CAD build for the part. Positions are in the model's coordinates, mm. Coordinates: 2 decimals unless noted, no trailing zeros. Loops run counter-clockwise (first coordinate to the right, second up) from the corner with the lowest first, then second, coordinate; pieces in that order, holes last. Notation, with made-up numbers: (65, 67) -> (84, 67) arc R30 cw to (84, 89) -> close; hole circle Ø3 at (30.25, 44.25). An arc over 180 degrees is marked (long way). Write each question's results on one line, items separated by ' | '.
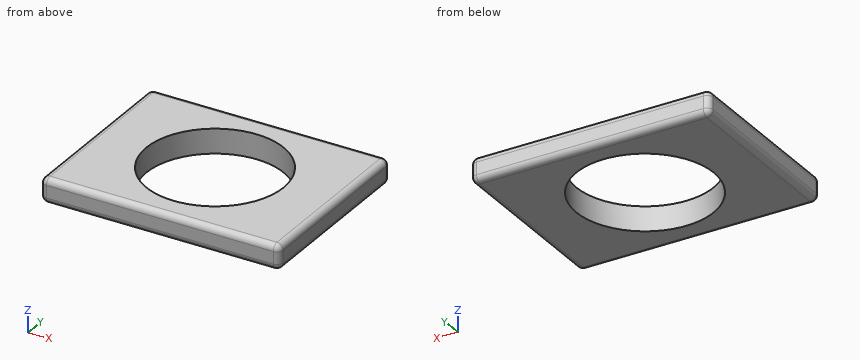
Autodesk Inventor part; units mm, degrees
ref_plane "YZ Plane" through (0, 0, 0) normal (1, 0, 0) x (0, 1, 0)
ref_plane "XZ Plane" through (0, 0, 0) normal (0, 1, 0) x (-1, 0, 0)
ref_plane "XY Plane" through (0, 0, 0) normal (0, 0, 1) x (1, 0, 0)
sketch "Sketch1" plane through (0, 0, 0) normal (0, 0, 1) x (1, 0, 0)
  line L0 (-9.75, -4.725) -> (-9.75, 4.725)
  line L1 (9.75, 4.725) -> (9.75, -4.725)
  circle A0 centre (0, 0) radius 5.6
  line L2 (0, 0) -> (0, 7.5)
  line L3 (0, 0) -> (0, -7.5)
  line L4 (-9.75, 7.5) -> (9.75, 7.5)
  line L5 (9.75, 7.5) -> (9.75, -7.5)
  line L6 (9.75, -7.5) -> (-9.75, -7.5)
  line L7 (-9.75, -7.5) -> (-9.75, 7.5)
  point P0 (0, 0)
  dimension "d0" = 11.2
  dimension "d5" = 7.5
  dimension "d6" = 7.5
extrude "Extrusion1" add sketch "Sketch1" along normal blind 2 contours L0 L7 L4 L2 A0 L3 L6 | L3 A0 L2 L4 L5 L1 L6
fillet "Fillet1" radius 0.5 4 edges at (9.75, 7.5, 1) (-9.75, 7.5, 1) (-9.75, -7.5, 1) (9.75, -7.5, 1)
fillet "Fillet2" radius 0.5 16 edges at (-9.6036, 7.3536, 2) (-9.75, 0, 2) (-9.6036, -7.3536, 2) (0, -7.5, 2) (9.6036, -7.3536, 2) (9.75, 0, 2) (9.6036, 7.3536, 2) (0, 7.5, 2) (9.6036, 7.3536, 0) (9.75, 0, 0) (9.6036, -7.3536, 0) (0, -7.5, 0) (-9.6036, -7.3536, 0) (-9.75, 0, 0) (-9.6036, 7.3536, 0) (0, 7.5, 0)
properties part number "SyringeAttachment"
Q1. Cut at C-C on z = 0.75. Write the cut outline in (x, y), and give its area (3 significant figures).
Results are:
outline: (-9.75, -7) arc R0.5 ccw to (-9.25, -7.5) -> (9.25, -7.5) arc R0.5 ccw to (9.75, -7) -> (9.75, 7) arc R0.5 ccw to (9.25, 7.5) -> (-9.25, 7.5) arc R0.5 ccw to (-9.75, 7) -> close; hole circle Ø11.2 at (0, 0) | area: 194 mm^2
Q2. Cut at B-B on y = 0. Write the cut outline in (x, z).
Results are:
outline: (-9.75, 0.5) arc R0.5 ccw to (-9.25, 0) -> (-5.6, 0) -> (-5.6, 2) -> (-9.25, 2) arc R0.5 ccw to (-9.75, 1.5) -> close; (5.6, 0) -> (9.25, 0) arc R0.5 ccw to (9.75, 0.5) -> (9.75, 1.5) arc R0.5 ccw to (9.25, 2) -> (5.6, 2) -> close
Q3. Wall check: L1, parallel to X at y = 0, z = 0.45; L2, parallel to Y at x = 0, z = 0.85. Give the ranges that are in metal, low to high. Write a range as from..to.
Results are:
L1: -9.75..-5.6, 5.6..9.75 | L2: -7.5..-5.6, 5.6..7.5
Q4. Cut at A-A on x = 0. Write the cut outline in (y, z), and give its area (3 significant figures).
Results are:
outline: (-7.5, 0.5) arc R0.5 ccw to (-7, 0) -> (-5.6, 0) -> (-5.6, 2) -> (-7, 2) arc R0.5 ccw to (-7.5, 1.5) -> close; (5.6, 0) -> (7, 0) arc R0.5 ccw to (7.5, 0.5) -> (7.5, 1.5) arc R0.5 ccw to (7, 2) -> (5.6, 2) -> close | area: 7.39 mm^2
